Check sheet for the drawn part. Datum: minimum x, y, z corner. Units: mm. A direction names the side the tool comes from. Coordinates: 2 decimals unless noted, no trailing zeros. Write each loop counter-clockwise with the first axis right and the second up, starting at its lowest first coordinate (ties: lowest second). Pieces come first, ordered by that corner, then holes. Notation, with made-up numbers: (-30.75, 4.5) -> (23.25, 4.5) arc R13 ccw to (23.25, 15.5) -> close; hole circle Ø9 at (-27.5, 12.5). An arc over 180 degrees is marked (long way). One line per question, with ' | ' between items.
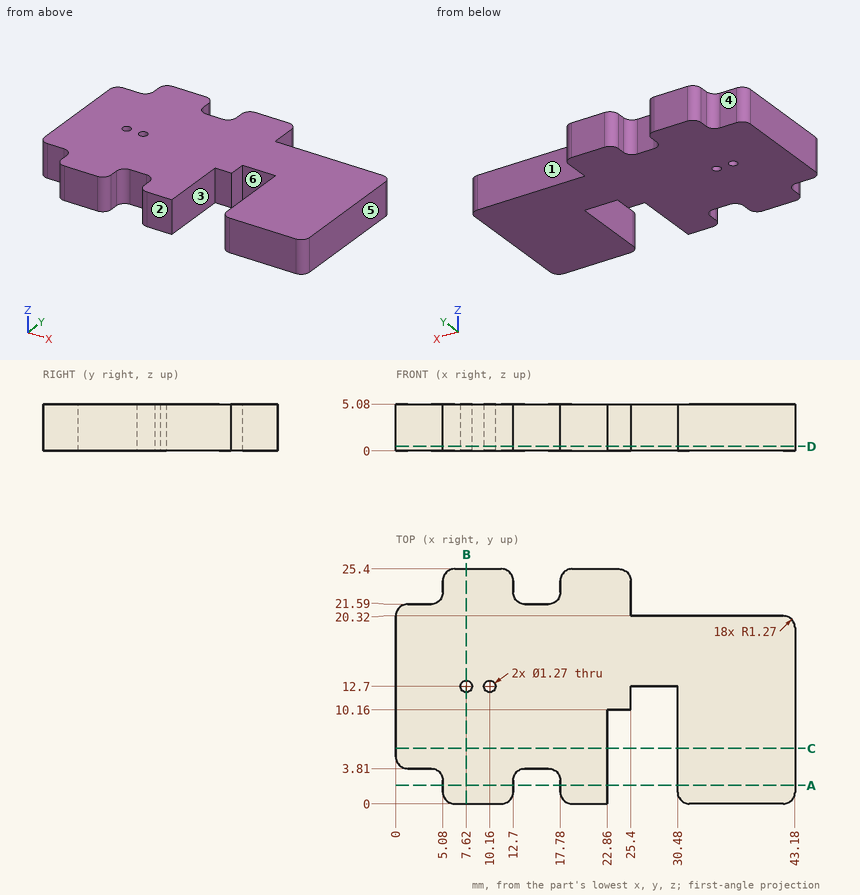
1. Go/stop test with flat-tipped pins: P1, Ø0.8, axis at x = 3, z = 3, coming from the -Y side; P2, Ø1.9, axis at y = 21.5, z = 2, coming from the +X side; P3, Ø1.3, axis at x = 15.5, z = 3.5, coming from the +Y side. Record where each tip stops, or that it passes through.
Worked answers:
P1: y = 3.81 | P2: x = 25.4 | P3: y = 21.59
2. Cross-section at B-B on x = 7.62. Record the boundary of the cut face in (y, z) (3 decimals).
Worked answers:
outline: (0, 0) -> (12.065, 0) -> (12.065, 5.08) -> (0, 5.08) -> close; (13.335, 0) -> (25.4, 0) -> (25.4, 5.08) -> (13.335, 5.08) -> close
3. Cross-section at A-A on y = 2. Record the boundary of the cut face in (x, z).
Worked answers:
outline: (5.08, 0) -> (12.7, 0) -> (12.7, 5.08) -> (5.08, 5.08) -> close; (17.78, 0) -> (22.86, 0) -> (22.86, 5.08) -> (17.78, 5.08) -> close; (30.48, 0) -> (43.18, 0) -> (43.18, 5.08) -> (30.48, 5.08) -> close
4. Cross-section at C-C on y = 6. Record the boundary of the cut face in (x, z), and give its area (3 significant figures).
Worked answers:
outline: (0, 0) -> (22.86, 0) -> (22.86, 5.08) -> (0, 5.08) -> close; (30.48, 0) -> (43.18, 0) -> (43.18, 5.08) -> (30.48, 5.08) -> close | area: 181 mm²
5. Mould release check, pull along X, two halves, no side actions. Record for the marked faces 4, 5 and 6: released by +X, released by -X, zero draft, split by the parting line, or undercut.
Worked answers:
face 4: zero draft | face 5: released by +X | face 6: undercut
6. Tool access check on the marked faces 1, 2 and 3. Record the directions out of +Z, -Z, +X, -X, +Y, -Y that give a thin tool (end or side, any length) a straight path to the whole face; none if there is none.
Worked answers:
face 1: +Z, -Z, +X, +Y | face 2: +Z, -Z, +X, -X, -Y | face 3: +Z, -Z, -Y
7. Cross-section at D-D on z = 0.5. Give the number of separate pieces and of enclosed holes in the cut face, and give its area (3 significant figures).
Worked answers:
separate pieces: 1 | enclosed holes: 2 | area: 834 mm²
8. Material ranges on line 1 (X direction, y = 2.5, z = 1.95); line 2 (Y direction, x = 7.62, z = 2.8) (3 decimals); line 3 (X direction, y = 13.25, z = 4.3), recorded low to high. Write a range as from..to.
Worked answers:
line 1: 5.08..12.7, 17.78..22.86, 30.48..43.18 | line 2: 0..12.065, 13.335..25.4 | line 3: 0..7.3, 7.94..9.84, 10.48..43.18
